Can you work these out from the model? Positions are in its coordinate system, mm. A direction names the side the tool comes from. Coordinates: 2 decimals unless noted, no trailing zeros. Order: outer loops, then holes, each group sorted by start corner. A loop starts at its lowest first (then second) coordinate and runs counter-clockwise, first axis right, second up. Notation, with made-up numbers: (66.5, 89.25) -> (123.5, 89.25) arc R15 ccw to (123.5, 95.25) -> close; hole circle Ø10 at (-11.5, -35.5). An arc over 180 degrees is marked (long way). Answer in a Markdown table with one row per item.
```python
from build123d import *

# Parameters (mm, degrees)
F0_R      = 31.75
F1_DEPTH  = 15
F2_SIZE   = 5
F3_R      = 25
F4_DEPTH  = 10
F5_SIZE2  = 9.99999
F5_SIZE   = 24.99999
F6_W      = 34.925
F6_H      = 17.4625
F7_DEPTH  = 104.774
F10_W     = 34.925
F10_H     = 34.925
F11_DEPTH = 34.925
F12_W     = 17.4625
F12_H     = 17.4625
F13_DEPTH = 17.4625
F14_DEPTH = 34.925
F15_W     = 17.4625
F15_H     = 17.4625
F15_H_2   = 34.925
F16_DEPTH = 17.4625
F19_W     = 8.73125
F19_H     = 8.73125
F20_DEPTH = 4.365625
F17_W     = 4.365625
F17_H     = 4.365625
F23_DEPTH = 4.365625
F24_DEPTH = 4.365625
F25_W     = 4.4006995887
F25_H     = 4.365625
F26_DEPTH = 4.365625
F27_DEPTH = 8.73125
F28_W     = 4.4006995887
F28_H     = 4.365625
F29_DEPTH = 4.365625
F30_W     = 4.4006995887
F30_H     = 4.365625
F31_DEPTH = 4.365625
F32_W     = 4.4006995887
F32_H     = 4.365
F33_DEPTH = 4.365625
F34_DEPTH = 8.73125
F35_W     = 4.4006995887
F35_H     = 4.365
F36_DEPTH = 4.365625
F37_DEPTH = 8.73125
F38_W     = 4.4006995887
F38_H     = 4.365
F39_DEPTH = 4.365625
F40_DEPTH = 8.73125
F42_W     = 4.365625
F42_H     = 4.365625
F43_DEPTH = 4.365625
F44_DEPTH = 4.365625
F46_DEPTH = 8.73125
F47_W     = 4.365625
F47_H     = 4.365625
F48_DEPTH = 25
F41_W     = 4.4006995887
F41_H     = 4.365
F49_DEPTH = 4.365625
F50_DEPTH = 8.73125
F51_W     = 4.4006995887
F51_H     = 4.365
F52_DEPTH = 4.365625
F53_DEPTH = 8.73215
F54_W     = 4.4006995887
F54_H     = 4.3659
F55_DEPTH = 4.365625
F56_DEPTH = 4.365625
F57_W     = 4.4006995887
F57_H     = 4.365625
F58_DEPTH = 4.365625
F59_W     = 4.4006995887
F59_H     = 8.73125
F60_DEPTH = 4.365625
F61_DEPTH = 4.365625
F62_DEPTH = 4.365625
F63_DEPTH = 4.365625
F64_W     = 4.4006995887
F64_H     = 8.73125
F65_DEPTH = 4.365625
F66_W     = 4.4006995887
F66_H     = 4.36625
F66_H_2   = 4.365625
F67_DEPTH = 4.365625
F68_W     = 4.4006995887
F68_H     = 4.365625
F69_DEPTH = 4.365625
F70_W     = 4.4006995887
F70_H     = 4.4238492846
F70_H_2   = 3.9164990911
F71_DEPTH = 4.3565625
F21_W     = 17.4625
F21_H     = 52.3875
F72_DEPTH = 4.365625


# Not quite as in the source:
# - a fillet or chamfer is up to 0.001 mm smaller than in the source, because OpenCascade refuses the exact size


with BuildPart() as f1:
    # F0 (on Top) → F1 (new body)
    with BuildSketch(Plane.XY):
        Circle(F0_R)
    extrude(amount=F1_DEPTH)

    # F2
    f2_edges = [f1.edges().sort_by_distance(p)[0] for p in [
        (-31.75, 0, 15),
    ]]
    chamfer(f2_edges, length=F2_SIZE)

    # F3 (on face) → F4 (cut)
    with BuildSketch(Plane(origin=(0, 0, 0), x_dir=(1, 0, 0), z_dir=(0, 0, -1))):
        Circle(F3_R)
    extrude(amount=-F4_DEPTH, mode=Mode.SUBTRACT)

    # F5 (size 25 and 10 in the source; OpenCascade refuses exactly that, so slightly less here)
    f5_edges = [f1.edges().sort_by_distance(p)[0] for p in [
        (-25, 0, 10),
    ]]
    f5_side = f1.faces().sort_by_distance((0, 0, 10))[0]
    chamfer(f5_edges, length=F5_SIZE, length2=F5_SIZE2, reference=f5_side)

    # F6 (on face) → F7 (join)
    with BuildSketch(Plane.XY.offset(15)):
        Rectangle(F6_W, F6_H)
    extrude(amount=F7_DEPTH)

    # F10 (on face) → F11 (join)
    with BuildSketch(Plane.XY.offset(119.774)):
        Rectangle(F10_W, F10_H)
    extrude(amount=F11_DEPTH)

    # F12 (on face) → F13 (join)
    with BuildSketch(Plane.YZ.offset(17.4625)):
        with Locations((0, 111.04275)):
            Rectangle(F12_W, F12_H)
    extrude(amount=F13_DEPTH)

    # F14 (add): a face of the model
    f14_faces = [f1.faces().sort_by_distance(p)[0] for p in [
        (26.19375, 0, 102.3115),
    ]]
    extrude(f14_faces, amount=F14_DEPTH)

    # F15 (on face) → F16 (join)
    with BuildSketch(Plane(origin=(-17.4625, 0, 0), x_dir=(0, -1, 0), z_dir=(-1, 0, 0))):
        with Locations((0, 111.04275)):
            Rectangle(F15_W, F15_H)
        with Locations((0, 84.849)):
            Rectangle(F15_W, F15_H_2)
    extrude(amount=F16_DEPTH)

    # F19 (on face) → F20 (cut)
    with BuildSketch(Plane.XZ.offset(17.4625)):
        Polygon((-8.73125, 127.5853067636), (-8.73125, 119.774), (-4.365625, 119.774), (-4.365625, 123.6796533818), (4.365625, 123.6796533818), (4.365625, 119.774), (8.73125, 119.774), (8.73125, 127.5853067636), (4.365625, 127.5853067636), (4.365625, 131.9509317636), (-4.365625, 131.9509317636), (-4.365625, 127.5853067636), align=None)
        with Locations((-8.068405883, 140.6821817636)):
            Rectangle(F19_W, F19_H)
        with Locations((8.73125, 140.6821817636)):
            Rectangle(F19_W, F19_H)
    extrude(amount=-F20_DEPTH, mode=Mode.SUBTRACT)

    # F17 (on face) → F23 (join)
    with BuildSketch(Plane(origin=(0, 8.73125, 0), x_dir=(-1, 0, 0), z_dir=(0, 1, 0))):
        with Locations((28.3765625, 69.5693125)):
            Rectangle(F17_W, F17_H)
    extrude(amount=F23_DEPTH)

    # F24 (add): a face of the model
    f24_faces = [f1.faces().sort_by_distance(p)[0] for p in [
        (-28.3765625, 10.9140625, 71.752125),
    ]]
    extrude(f24_faces, amount=F24_DEPTH)

    # F25 (on face) → F26 (join)
    with BuildSketch(Plane.XZ.offset(8.73125)):
        with Locations((-28.3590252057, 69.5693125)):
            Rectangle(F25_W, F25_H)
    extrude(amount=F26_DEPTH)

    # F27 (add): a face of the model
    f27_faces = [f1.faces().sort_by_distance(p)[0] for p in [
        (-28.3590252057, -10.9140625, 71.752125),
    ]]
    extrude(f27_faces, amount=F27_DEPTH)

    # F28 (on face) → F29 (join)
    with BuildSketch(Plane.XZ.offset(13.096875)):
        with Locations((-28.3590252057, 73.9349375)):
            Rectangle(F28_W, F28_H)
        with Locations((-28.3590252057, 78.3005625)):
            Rectangle(F28_W, F28_H)
    extrude(amount=F29_DEPTH)

    # F30 (on face) → F31 (join)
    with BuildSketch(Plane.XY.offset(80.483375)):
        with Locations((-28.3590252057, -15.2796875)):
            Rectangle(F30_W, F30_H)
    extrude(amount=F31_DEPTH)

    # F32 (on face) → F33 (join)
    with BuildSketch(Plane.XZ.offset(17.4625)):
        with Locations((-28.3590252057, 78.300875)):
            Rectangle(F32_W, F32_H)
    extrude(amount=F33_DEPTH)

    # F34 (add): a face of the model
    f34_faces = [f1.faces().sort_by_distance(p)[0] for p in [
        (-28.3590252057, -19.6453125, 80.483375),
    ]]
    extrude(f34_faces, amount=F34_DEPTH)

    # F35 (on face) → F36 (join)
    with BuildSketch(Plane.XZ.offset(21.828125)):
        with Locations((-28.3590252057, 82.6665)):
            Rectangle(F35_W, F35_H)
    extrude(amount=F36_DEPTH)

    # F37 (add): a face of the model
    f37_faces = [f1.faces().sort_by_distance(p)[0] for p in [
        (-28.3590252057, -24.0109375, 84.849),
    ]]
    extrude(f37_faces, amount=F37_DEPTH)

    # F38 (on face) → F39 (join)
    with BuildSketch(Plane.XZ.offset(26.19375)):
        with Locations((-28.3590252057, 87.032125)):
            Rectangle(F38_W, F38_H)
    extrude(amount=F39_DEPTH)

    # F40 (add): a face of the model
    f40_faces = [f1.faces().sort_by_distance(p)[0] for p in [
        (-28.3590252057, -28.3765625, 89.214625),
    ]]
    extrude(f40_faces, amount=F40_DEPTH)

    # F42 (on face) → F43 (cut)
    with BuildSketch(Plane(origin=(0, 13.096875, 0), x_dir=(-1, 0, 0), z_dir=(0, 1, 0))):
        with Locations((28.3765625, 73.9349375)):
            Rectangle(F42_W, F42_H)
    extrude(amount=-F43_DEPTH, mode=Mode.SUBTRACT)

    # F44 (add): a face of the model
    f44_faces = [f1.faces().sort_by_distance(p)[0] for p in [
        (-28.3765625, 13.096875, 69.5693125),
    ]]
    extrude(f44_faces, amount=F44_DEPTH)

    # F45 (on face) → F46 (join)
    with BuildSketch(Plane(origin=(0, 0, 67.3865), x_dir=(1, 0, 0), z_dir=(0, 0, -1))):
        Polygon((-30.559375, -4.365625), (-30.559375, -8.73125), (-30.559375, -17.4625), (-26.19375, -17.4625), (-26.19375, -8.73125), (-26.19375, -4.365625), align=None)
    extrude(amount=F46_DEPTH)

    # F47 (on face) → F48 (cut)
    with BuildSketch(Plane(origin=(-30.559375, 0, 0), x_dir=(0, -1, 0), z_dir=(-1, 0, 0))):
        with Locations((-10.9140625, 65.2036875)):
            Rectangle(F47_W, F47_H)
    extrude(amount=-F48_DEPTH, mode=Mode.SUBTRACT)

    # F41 (on face) → F49 (join)
    with BuildSketch(Plane.XZ.offset(30.559375)):
        with Locations((-28.3590252057, 91.39775)):
            Rectangle(F41_W, F41_H)
    extrude(amount=F49_DEPTH)

    # F50 (add): a face of the model
    f50_faces = [f1.faces().sort_by_distance(p)[0] for p in [
        (-28.3590252057, -32.7421875, 93.58025),
    ]]
    extrude(f50_faces, amount=F50_DEPTH)

    # F51 (on face) → F52 (join)
    with BuildSketch(Plane.XZ.offset(34.925)):
        with Locations((-28.3590252057, 95.763375)):
            Rectangle(F51_W, F51_H)
    extrude(amount=F52_DEPTH)

    # F53 (add): a face of the model
    f53_faces = [f1.faces().sort_by_distance(p)[0] for p in [
        (-28.3590252057, -37.1078125, 97.945875),
    ]]
    extrude(f53_faces, amount=F53_DEPTH)

    # F54 (on face) → F55 (join)
    with BuildSketch(Plane.XZ.offset(39.290625)):
        with Locations((-28.3590252057, 100.12945)):
            Rectangle(F54_W, F54_H)
    extrude(amount=F55_DEPTH)

    # F56 (add): a face of the model
    f56_faces = [f1.faces().sort_by_distance(p)[0] for p in [
        (-28.3590252057, -41.4734375, 102.3124),
    ]]
    extrude(f56_faces, amount=F56_DEPTH)

    # F57 (on face) → F58 (join)
    with BuildSketch(Plane.XZ.offset(43.65625)):
        with Locations((-28.3590252057, 104.4952125)):
            Rectangle(F57_W, F57_H)
    extrude(amount=F58_DEPTH)

    # F59 (on face) → F60 (join)
    with BuildSketch(Plane.XY.offset(106.678025)):
        with Locations((-28.3590252057, -43.65625)):
            Rectangle(F59_W, F59_H)
    extrude(amount=F60_DEPTH)

    # F61 (add): faces of the model
    f61_faces = [f1.faces().sort_by_distance(p)[0] for p in [
        (-28.3590252057, -10.9140625, 80.483375),
        (-28.3590252057, -15.2796875, 84.849),
        (-28.3590252057, -19.6453125, 89.214625),
        (-28.3590252057, -24.0109375, 93.58025),
        (-28.3590252057, -28.3765625, 97.945875),
        (-28.3590252057, -32.7421875, 102.3115),
        (-28.3590252057, -37.1078125, 106.678025),
        (-28.3590252057, -43.65625, 111.04365),
    ]]
    extrude(f61_faces, amount=F61_DEPTH)

    # F62 (add): faces of the model
    f62_faces = [f1.faces().sort_by_distance(p)[0] for p in [
        (-28.3590252057, -10.9140625, 84.849),
        (-28.3590252057, -15.2796875, 89.214625),
        (-28.3590252057, -19.6453125, 93.58025),
        (-28.3590252057, -24.0109375, 97.945875),
        (-28.3590252057, -28.3765625, 102.3115),
        (-28.3590252057, -32.7421875, 106.677125),
        (-28.3590252057, -37.1078125, 111.04365),
    ]]
    extrude(f62_faces, amount=F62_DEPTH)

    # F63 (add): a face of the model
    f63_faces = [f1.faces().sort_by_distance(p)[0] for p in [
        (-28.3590252057, -15.2796875, 71.752125),
    ]]
    extrude(f63_faces, amount=F63_DEPTH)

    # F64 (on face) → F65 (join)
    with BuildSketch(Plane(origin=(0, 0, 67.3865), x_dir=(1, 0, 0), z_dir=(0, 0, -1))):
        with Locations((-28.3590252057, 13.096875)):
            Rectangle(F64_W, F64_H)
    extrude(amount=F65_DEPTH)

    # F66 (on face) → F67 (join)
    with BuildSketch(Plane.XZ.offset(17.4625)):
        with Locations((-28.3590252057, 69.569625)):
            Rectangle(F66_W, F66_H)
        with Locations((-28.3590252057, 65.2036875)):
            Rectangle(F66_W, F66_H_2)
    extrude(amount=F67_DEPTH)

    # F68 (on face) → F69 (join)
    with BuildSketch(Plane(origin=(0, 0, 63.020875), x_dir=(1, 0, 0), z_dir=(0, 0, -1))):
        with Locations((-28.3590252057, 19.6453125)):
            Rectangle(F68_W, F68_H)
    extrude(amount=F69_DEPTH)

    # F70 (on face) → F71 (join)
    with BuildSketch(Plane.XZ.offset(21.828125)):
        with Locations((-28.3590252057, 64.7836737335)):
            Rectangle(F70_W, F70_H)
        with Locations((-28.3590252057, 60.6134995456)):
            Rectangle(F70_W, F70_H_2)
    extrude(amount=F71_DEPTH)

    # F21 (on face) → F72 (cut)
    with BuildSketch(Plane.XZ.offset(8.73125)):
        with Locations((0, 93.58025)):
            Rectangle(F21_W, F21_H)
    extrude(amount=-F72_DEPTH, mode=Mode.SUBTRACT)


solid = f1.part
```
(1) On a 3-axis mill with a long thin cutter (end or side, diameter ignored), from which of +Z, -Z, +X, -X, +Y, -Y can I reach the whole of each face in a straight line? I mean faces 4 (the flat face through (-28, -28, 106.677)), 5 (the flat face through (-28, -24, 80.484)), 6 (the flat face through (4.366, -15, 122)), 7 (the flat face through (-28, -33, 89.215)), 8 (the conical face through (-21.42, -16.42, 14.76)). Say none if no direction works.
Response values:
| item | result |
|---|---|
| face 4 | +Z, +X, -X |
| face 5 | +X, -X, -Y |
| face 6 | -Y |
| face 7 | -Z, +X, -X, -Y |
| face 8 | none |
(2) Will these pins go through, and if not, where does the flat tip stop? pin 1 Ø5 at (x, z) = (-28.5, 65.5) entering from +Y; pin 2 Ø7 at (x, z) = (-8, 141.5) entering from -Y; pin 3 Ø1.5 at (x, z) = (-15.5, 105.5) entering from -Y.
Response values:
| item | result |
|---|---|
| pin 1 | y = 17.46 |
| pin 2 | y = -13.1 |
| pin 3 | y = -8.73 |
(3) We'd pull the mould along Z, two halves only. Please class faces 1 (the flat face through (-28, -26.194, 83)), 2 (the flat face through (-3.703, -15, 141)), 3 (the flat face through (26, 0, 119.774)): +Z half, -Z half, draft (parallel to the pull), parting line (faces both ways), or undercut.
Response values:
| item | result |
|---|---|
| face 1 | draft |
| face 2 | undercut |
| face 3 | +Z half |
(4) Suppose I cut it at A-A (z = 47.5). Please give me the cut outline in (x, y), and give its area (3 significant figures).
Response values:
| item | result |
|---|---|
| outline | (-17.46, -8.73) -> (17.46, -8.73) -> (17.46, 8.73) -> (-17.46, 8.73) -> close |
| area | 610 mm2 |
(5) I need wall thicknesses on line 1 (Z direction, x = -26, y = -1); line 2 (X direction, y = -17, z = 127); line 3 (Z direction, x = -29.5, y = 13.5). Which ranges of each line are inside material? Lowest first, please. Write a range as [from, to].
Response values:
| item | result |
|---|---|
| line 1 | [0, 15], [67.39, 119.77] |
| line 2 | [-17.46, -8.73], [8.73, 17.46] |
| line 3 | [58.66, 71.75] |
